CAD build for the part. Positions are in the model's coordinates, mm. Face numbers are marked on the shaded views. A direction names the side the tool comes from. Give positions to 0.01 mm unless a question says otherwise; leave off trailing zeros. Write each loop counter-clockwise with the first axis right and the second up, starting at its lowest first coordinate (ties: lowest second). Pieces come first, ordered by that corner, then holes. Notation, with made-up numbers: (82.25, -30.5) - (91.25, -30.5) arc R21 cw to (91.25, -26.5) - close; hole circle Ø2 at (55.5, 56). An arc over 180 degrees is marked (long way). Answer as a JSON object with one key per item and string values.
from build123d import *

# Parameters (mm, degrees)
SKETCH1_R                    = 6.5
BASE_FLANGE1_DEPTH           = 3.175
EDGE_FLANGE1_STRIP_W         = 14.1732
EDGE_FLANGE1_STRIP_H         = 3.175
EDGE_FLANGE1_STRIP_CUT_DEPTH = 50
EDGE_FLANGE1_DEPTH           = 50
FILLET2_R                    = 2


# Sheet-metal steps are written as plain solids
with BuildPart() as part:
    # Sketch1 → Base-Flange1 (new body)
    with BuildSketch(Plane.XY):
        with BuildLine():
            Line((-25, 0), (25, 0))
            Line((25, 0), (25, 1.175))
            ThreePointArc((25, 1.175), (24.414213562, 2.589213562), (23, 3.175))
            Line((23, 3.175), (14, 3.175))
            ThreePointArc((14, 3.175), (12.585786438, 3.760786438), (12, 5.175))
            Line((12, 5.175), (12, 13.175))
            ThreePointArc((12, 13.175), (0, 25.175), (-12, 13.175))
            Line((-12, 13.175), (-12, 5.175))
            ThreePointArc((-12, 5.175), (-12.585786438, 3.760786438), (-14, 3.175))
            Line((-14, 3.175), (-23, 3.175))
            ThreePointArc((-23, 3.175), (-24.414213562, 2.589213562), (-25, 1.175))
            Line((-25, 1.175), (-25, 0))
        make_face()
        with Locations((0, 13.175)):
            Circle(SKETCH1_R, mode=Mode.SUBTRACT)
    extrude(amount=-BASE_FLANGE1_DEPTH)

    # Edge-Flange1 strip (across the edge) → Edge-Flange1 strip cut (cut)
    with BuildSketch(Plane(origin=(25, 0, -3.175), x_dir=(0, 1, 0), z_dir=(-1, 0, 0))):
        with Locations((-6.35, -1.5875)):
            Rectangle(EDGE_FLANGE1_STRIP_W, EDGE_FLANGE1_STRIP_H)
    extrude(amount=EDGE_FLANGE1_STRIP_CUT_DEPTH, mode=Mode.SUBTRACT)

    # Edge-Flange1 section (across the edge) → Edge-Flange1 (add)
    with BuildSketch(Plane(origin=(25, 0, -3.175), x_dir=(0, 1, 0), z_dir=(-1, 0, 0))):
        with BuildLine():
            Line((-3.175, 0.7366), (-3.175, 16.825))
            Line((-3.175, 16.825), (0, 16.825))
            Line((0, 16.825), (0, 0.7366))
            ThreePointArc((0, 0.7366), (0.215745145, 0.215745145), (0.7366, 0))
            Line((0.7366, 0), (0.7366, -3.175))
            ThreePointArc((0.7366, -3.175), (-2.029318885, -2.029318885), (-3.175, 0.7366))
        make_face()
    extrude(amount=EDGE_FLANGE1_DEPTH)

    # Fillet2
    fillet2_edges = [part.edges().sort_by_distance(p)[0] for p in [
        (25, -1.5875, -20),
        (-25, -1.5875, -20),
    ]]
    fillet(fillet2_edges, radius=FILLET2_R)


solid = part.part
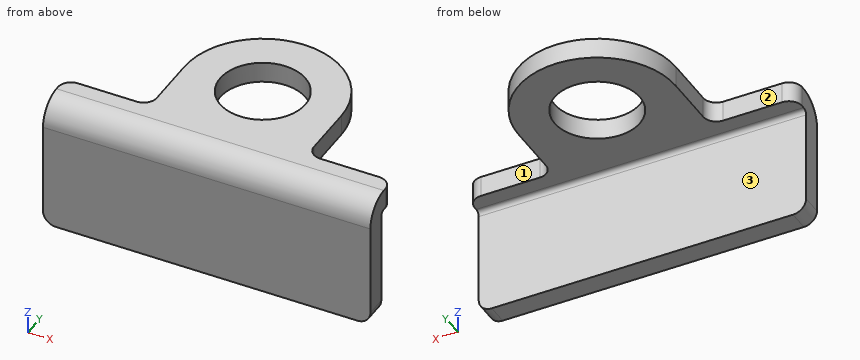
(1) Saw through at C-C, the plane z = -10. Give the cut face in (x, y) (3 decimals), and give its area (3 significant figures).
Answer key:
{"outline": "(-25, -3.175) - (25, -3.175) - (25, 0) - (-25, 0) - close", "area": "159 mm²"}
(2) Saw through at D-D, the plane x = 9.5. Give the cut face in (y, z) (3 decimals).
Answer key:
{"outline": "(-3.175, -20) - (0, -20) - (0, -3.912) arc R0.737 cw to (0.737, -3.175) - (20.506, -3.175) - (20.506, 0) - (0.737, 0) arc R3.912 ccw to (-3.175, -3.912) - close"}
(3) Probe L1, parallel to Z at x = 9.5, y = 8.75 (3 decimals); L2, parallel to Y at x = 0, z = -0.75 (3 decimals). List the from-to ranges inside material, lowest first. Write a range as [from, to].
Answer key:
{"L1": "z = [-3.175, 0]", "L2": "y = [-1.567, 6.675], [19.675, 25.175]"}
(4) Flat gauge pins, fed straight in: P1, Ø12, axis at y = 11, z = -3, coming from the +X side; P2, Ø8, axis at x = 1.5, y = 16.5, coming from the -Z side (3 decimals); P3, Ø1, axis at x = 20.5, z = -2, coming from the +Y side (3 decimals). Where does each tip first touch, or does it go through?
Answer key:
{"P1": "stops at x = 12.01", "P2": "stops at z = -3.175", "P3": "stops at y = 3.175"}
(5) Saw through at A-A, the plane x = 0. Give the cut face in (y, z) (3 decimals).
Answer key:
{"outline": "(-3.175, -20) - (0, -20) - (0, -3.912) arc R0.737 cw to (0.737, -3.175) - (6.675, -3.175) - (6.675, 0) - (0.737, 0) arc R3.912 ccw to (-3.175, -3.912) - close; (19.675, -3.175) - (25.175, -3.175) - (25.175, 0) - (19.675, 0) - close"}
(6) Saw through at B-B, the plane y = 11. Give the cut face in (x, z) (3 decimals), and give its area (3 significant figures).
Answer key:
{"outline": "(-12, -3.175) - (-6.125, -3.175) - (-6.125, 0) - (-12, 0) - close; (6.125, -3.175) - (12, -3.175) - (12, 0) - (6.125, 0) - close", "area": "37.3 mm²"}
(7) 3-axis set-ups, long thin cutter, end or side, ignore diameter. For the marked faces 1, 2 and 3: which of +Z, -Z, +X, -X, +Y, -Y reach the whole face in a straight line?
Answer key:
{"face 1": "+Z, -Z, +X, +Y", "face 2": "+Z, -Z, -X, +Y", "face 3": "-Z, +X, -X, +Y"}
